Input: part model. Units: mm. Frame: model coordinates. A direction names the side the tool comes from. Round coordinates to 2 decimals unless told otherwise and drop trailing zeros. Order: outer loops, then holes, each group sorted by start corner. A loop starts at its lowest first (then second) coordinate and runs counter-clockwise, first axis right, second up. Notation, with made-up numbers: M 55.25,62 L 83.25,62 A20 cw 83.25,98 Z; hole C -26,21 d7. An arc over 180 degrees is marked long. One line per question, with ' | ' between items.
```python
from build123d import *

# Parameters (mm, degrees)
SKETCH1_R               = 12.7
BOSS_EXTRUDE1_DEPTH     = 5
SKETCH2_R               = 6
BOSS_EXTRUDE2_DEPTH     = 4.2
CUT_EXTRUDE1_REACH      = 20.643
SKETCH3_R               = 1.425
CUT_EXTRUDE2_DEPTH      = 21.179692763
CUT_EXTRUDE2_DEPTH_BACK = 21.179692763
SKETCH4_R               = 3


with BuildPart() as part:
    # Sketch1 → Boss-Extrude1 (new body)
    with BuildSketch(Plane.XY):
        Circle(SKETCH1_R)
    extrude(amount=BOSS_EXTRUDE1_DEPTH)

    # Sketch2 → Boss-Extrude2 (add)
    with BuildSketch(Plane.XY.offset(5)):
        Circle(SKETCH2_R)
    extrude(amount=BOSS_EXTRUDE2_DEPTH)

    # Sketch3 → Cut-Extrude1 (cut, up to next)
    with BuildSketch(Plane.XY.offset(5), mode=Mode.PRIVATE) as cut_extrude1_sk1:
        with Locations((0, 9.5)):
            Circle(SKETCH3_R)
    cut_extrude1_tool1 = extrude(cut_extrude1_sk1.sketch, amount=-CUT_EXTRUDE1_REACH, mode=Mode.PRIVATE) & part.part
    # Sketch3 → Cut-Extrude1 (cut, up to next)
    with BuildSketch(Plane.XY.offset(5), mode=Mode.PRIVATE) as cut_extrude1_sk2:
        with Locations((-8.227241336, 4.75)):
            Circle(SKETCH3_R)
    cut_extrude1_tool2 = extrude(cut_extrude1_sk2.sketch, amount=-CUT_EXTRUDE1_REACH, mode=Mode.PRIVATE) & part.part
    # Sketch3 → Cut-Extrude1 (cut, up to next)
    with BuildSketch(Plane.XY.offset(5), mode=Mode.PRIVATE) as cut_extrude1_sk3:
        with Locations((-8.227241336, -4.75)):
            Circle(SKETCH3_R)
    cut_extrude1_tool3 = extrude(cut_extrude1_sk3.sketch, amount=-CUT_EXTRUDE1_REACH, mode=Mode.PRIVATE) & part.part
    # Sketch3 → Cut-Extrude1 (cut, up to next)
    with BuildSketch(Plane.XY.offset(5), mode=Mode.PRIVATE) as cut_extrude1_sk4:
        with Locations((0, -9.5)):
            Circle(SKETCH3_R)
    cut_extrude1_tool4 = extrude(cut_extrude1_sk4.sketch, amount=-CUT_EXTRUDE1_REACH, mode=Mode.PRIVATE) & part.part
    # Sketch3 → Cut-Extrude1 (cut, up to next)
    with BuildSketch(Plane.XY.offset(5), mode=Mode.PRIVATE) as cut_extrude1_sk5:
        with Locations((8.227241336, -4.75)):
            Circle(SKETCH3_R)
    cut_extrude1_tool5 = extrude(cut_extrude1_sk5.sketch, amount=-CUT_EXTRUDE1_REACH, mode=Mode.PRIVATE) & part.part
    # Sketch3 → Cut-Extrude1 (cut, up to next)
    with BuildSketch(Plane.XY.offset(5), mode=Mode.PRIVATE) as cut_extrude1_sk6:
        with Locations((8.227241336, 4.75)):
            Circle(SKETCH3_R)
    cut_extrude1_tool6 = extrude(cut_extrude1_sk6.sketch, amount=-CUT_EXTRUDE1_REACH, mode=Mode.PRIVATE) & part.part
    add(cut_extrude1_tool1.solids().sort_by_distance((0, 9.5, 5))[0], mode=Mode.SUBTRACT)
    add(cut_extrude1_tool2.solids().sort_by_distance((-8.227241, 4.75, 5))[0], mode=Mode.SUBTRACT)
    add(cut_extrude1_tool3.solids().sort_by_distance((-8.227241, -4.75, 5))[0], mode=Mode.SUBTRACT)
    add(cut_extrude1_tool4.solids().sort_by_distance((0, -9.5, 5))[0], mode=Mode.SUBTRACT)
    add(cut_extrude1_tool5.solids().sort_by_distance((8.227241, -4.75, 5))[0], mode=Mode.SUBTRACT)
    add(cut_extrude1_tool6.solids().sort_by_distance((8.227241, 4.75, 5))[0], mode=Mode.SUBTRACT)

    # Sketch4 → Cut-Extrude2 (cut, two sides: drawn at the far end of the back side and taken through both)
    with BuildSketch(Plane.XY.offset(9.2).offset(-CUT_EXTRUDE2_DEPTH_BACK)):
        Circle(SKETCH4_R)
    extrude(amount=CUT_EXTRUDE2_DEPTH + CUT_EXTRUDE2_DEPTH_BACK, mode=Mode.SUBTRACT)


solid = part.part
```
Item 1: Section query B-B, the plane y = 0. Return loops of the section in (x, z).
Report:
outline: M -12.7,0 L -3,0 L -3,9.2 L -6,9.2 L -6,5 L -12.7,5 Z; M 3,0 L 12.7,0 L 12.7,5 L 6,5 L 6,9.2 L 3,9.2 Z
Item 2: Section query A-A, the plane x = 0. Return loops of the section in (y, z) (3 decimals), plus the area to 3 significant figures.
Report:
outline: M -12.7,0 L -10.925,0 L -10.925,5 L -12.7,5 Z; M -8.075,0 L -3,0 L -3,9.2 L -6,9.2 L -6,5 L -8.075,5 Z; M 3,0 L 8.075,0 L 8.075,5 L 6,5 L 6,9.2 L 3,9.2 Z; M 10.925,0 L 12.7,0 L 12.7,5 L 10.925,5 Z | area: 93.7 mm²
Item 3: Access query for faces 1 (the flat face through (5.5, 3, 5)), 2 (the cylindrical face through (0.658, 8.236, 2.535)). Directions: +Z, -Z, +X, -X, +Y, -Y. A direction counts if a zero-diameter tool reaches every point of the face in a straight line with its end or side. Return the directions, or none.
Report:
face 1: +Z | face 2: +Z, -Z
Item 4: First-contact query: pin 1 (8 mm diameter, centred on x = 3.5, y = -9.5, fed in from +Z); pin 2 (1 mm diameter, centred on x = 1, z = 3, fed in from -Y); pin 3 (1.5 mm diameter, centred on y = -7, z = 3.5, fed in from -X). Flat tips, straight axial feed; report the tip coordinate or a pass-through.
Report:
pin 1: z = 5 | pin 2: y = -12.69 | pin 3: x = -11.06
Item 5: Section query C-C, the plane z = 3.75. Return loops of the section in (x, y) (3 decimals).
Report:
outline: C 0,0 d25.4; hole C -8.227,-4.75 d2.85; hole C -8.227,4.75 d2.85; hole C 0,0 d6; hole C 0,-9.5 d2.85; hole C 0,9.5 d2.85; hole C 8.227,-4.75 d2.85; hole C 8.227,4.75 d2.85
Item 6: Line query: line 1 along Y through (x, z) = (0, 1.55) (3 decimals); line 2 along X through (y, z) = (-5, 1.25); line 3 along Z through (x, y) = (-7, -6.5). Output: solid intervals per line, ascending. Write a range as from..to.
Report:
line 1: -12.7..-10.925, -8.075..-3, 3..8.075, 10.925..12.7 | line 2: -11.67..-9.63, -6.82..6.82, 9.63..11.67 | line 3: 0..5
Item 7: Section query D-D, the plane y = 4.75. Return loops of the section in (x, z).
Report:
outline: M -11.78,0 L -9.65,0 L -9.65,5 L -11.78,5 Z; M -6.8,0 L 6.8,0 L 6.8,5 L 3.67,5 L 3.67,9.2 L -3.67,9.2 L -3.67,5 L -6.8,5 Z; M 9.65,0 L 11.78,0 L 11.78,5 L 9.65,5 Z
Item 8: Mould query, pull axis X, two halves, no side actions, for faces 3 (the flat face through (-3, -1, 9.2)), 4 (the cylindrical face through (0.77, -8.3, 2.54)), 5 (the cylindrical face through (-6, 0, 7)). Classes: +X half, -X half, draft (parallel to the pull), parting line (faces both ways), or undercut.
Report:
face 3: draft | face 4: undercut | face 5: parting line
